Could you check a few things on this model? Use its own coordinates, in mm. Face numbers are marked on the shaded views. Round coordinates to 2 decimals unless told otherwise and drop trailing zeros. Write each loop counter-clockwise with the first axis right and the second up, starting at its lowest first coordinate (ties: lowest second). Pieces come first, ordered by that corner, then holes. Notation, with made-up numbers: M -14,81 L 7,81 A20 ccw 7,96 Z; hole C 12.25,-17 d8. An arc over 180 degrees is marked long. One line per question, with ' | ' between items. Start each with the question number.
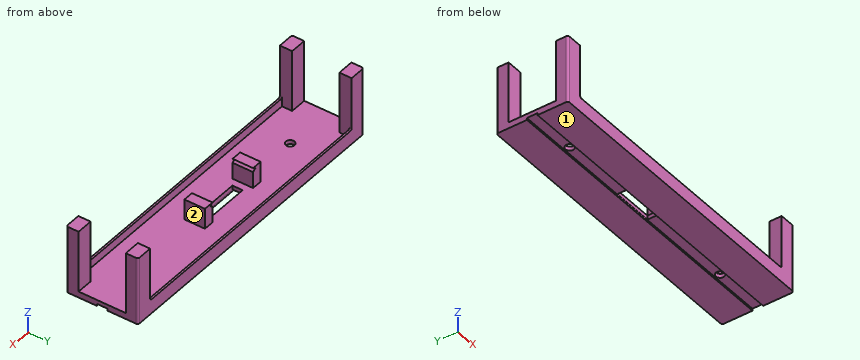
```python
from build123d import *

# Parameters (mm, degrees)
SKICA1_W                 = 150
SKICA1_H                 = 35
P_IDAT_VYSUNUT_M2_DEPTH  = 3
SKICA4_W                 = 20
SKICA4_H                 = 5
ODEBRAT_VYSUNUT_M1_DEPTH = 2
SKICA5_W                 = 150
SKICA5_H                 = 5.2
ODEBRAT_VYSUNUT_M3_DEPTH = 1
SKICA7_R                 = 2.1
ODEBRAT_VYSUNUT_M4_DEPTH = 3
SKICA8_W                 = 8
SKICA8_H                 = 6
P_IDAT_VYSUNUT_M4_DEPTH  = 30
ZAOBLIT1_R               = 1
SKICA9_W                 = 134
SKICA9_H                 = 1
P_IDAT_VYSUNUT_M5_DEPTH  = 4
ZAOBLIT2_R               = 1
SKICA10_W                = 5
SKICA10_H                = 10
P_IDAT_VYSUNUT_M6_DEPTH  = 10
ODEBRAT_VYSUNUT_M6_DEPTH = 10


with BuildPart() as part:
    # Skica1 → Přidat vysunutím2 (new body)
    with BuildSketch(Plane.XY):
        Rectangle(SKICA1_W, SKICA1_H)
    extrude(amount=P_IDAT_VYSUNUT_M2_DEPTH)

    # Skica4 → Odebrat vysunutím1 (cut)
    with BuildSketch(Plane.XY.offset(3)):
        with Locations((-5, 0)):
            Rectangle(SKICA4_W, SKICA4_H)
    extrude(amount=-ODEBRAT_VYSUNUT_M1_DEPTH, mode=Mode.SUBTRACT)

    # Skica5 → Odebrat vysunutím3 (cut)
    with BuildSketch(Plane(origin=(0, 0, 0), x_dir=(-1, 0, 0), z_dir=(0, 0, -1))):
        Rectangle(SKICA5_W, SKICA5_H)
    extrude(amount=-ODEBRAT_VYSUNUT_M3_DEPTH, mode=Mode.SUBTRACT)

    # Skica7 → Odebrat vysunutím4 (cut, through all)
    with BuildSketch(Plane(origin=(0, 0, 1), x_dir=(-1, 0, 0), z_dir=(0, 0, -1))):
        with Locations((-50, 0)):
            Circle(SKICA7_R)
        with Locations((50, 0)):
            Circle(SKICA7_R)
    extrude(amount=-ODEBRAT_VYSUNUT_M4_DEPTH, mode=Mode.SUBTRACT)

    # Skica8 → Přidat vysunutím4 (add)
    with BuildSketch(Plane.XY.offset(3)):
        with Locations((71, 14.5)):
            Rectangle(SKICA8_W, SKICA8_H)
        with Locations((71, -14.5)):
            Rectangle(SKICA8_W, SKICA8_H)
        with Locations((-71, -14.5)):
            Rectangle(SKICA8_W, SKICA8_H)
        with Locations((-71, 14.5)):
            Rectangle(SKICA8_W, SKICA8_H)
    extrude(amount=P_IDAT_VYSUNUT_M4_DEPTH)

    # Zaoblit1
    zaoblit1_edges = [part.edges().sort_by_distance(p)[0] for p in [
        (75, -17.5, 16.5),
        (75, 17.5, 16.5),
        (-75, 17.5, 16.5),
        (-75, -17.5, 16.5),
    ]]
    fillet(zaoblit1_edges, radius=ZAOBLIT1_R)

    # Skica9 → Přidat vysunutím5 (add)
    with BuildSketch(Plane.XY.offset(3)):
        with Locations((0, 17)):
            Rectangle(SKICA9_W, SKICA9_H)
        with Locations((0, -17)):
            Rectangle(SKICA9_W, SKICA9_H)
    extrude(amount=P_IDAT_VYSUNUT_M5_DEPTH)

    # Zaoblit2
    zaoblit2_edges = [part.edges().sort_by_distance(p)[0] for p in [
        (67, 17, 7),
        (-67, 17, 7),
        (-67, -17, 7),
        (67, -17, 7),
    ]]
    fillet(zaoblit2_edges, radius=ZAOBLIT2_R)

    # Skica10 → Přidat vysunutím6 (add)
    with BuildSketch(Plane.XY.offset(3)):
        with Locations((-21, 0)):
            Rectangle(SKICA10_W, SKICA10_H)
        with Locations((11, 0)):
            Rectangle(SKICA10_W, SKICA10_H)
    extrude(amount=P_IDAT_VYSUNUT_M6_DEPTH)

    # Skica12 → Odebrat vysunutím6 (cut)
    with BuildSketch(Plane(origin=(0, 5, 0), x_dir=(1, 0, 0), z_dir=(0, 1, 0))):
        Polygon((-18.5, -13), (-18.5, -11), (-20, -12), align=None)
        Polygon((8.5, -13), (8.5, -11), (10, -12), align=None)
    extrude(amount=-ODEBRAT_VYSUNUT_M6_DEPTH, mode=Mode.SUBTRACT)


solid = part.part
```
1. Suppose I cut it at B-B (x = -50). Write out the boundary of the cut face in (y, z), and give its area (3 significant figures).
2. Suppose I cut it at A-A (z = 20.5). Write out the boundary of the cut face in (x, y), and give its area (3 significant figures).
3. I'm going to push flat-ended pins straight in: P1, Ø4, axis at y = -2, z = 6.5, coming from the +X side; P2, Ø3, axis at x = 12.5, z = 10.5, coming from the -Y side; P3, Ø16.5, axis at x = 32, y = -4.5, coming from the +Z side. Where does each tip first touch, or does it pass through?
4. If we mould it in two halves opening along Y, with no side actions, what happens to the marked faces 1 and 2? For each: released by +Y, released by -Y, zero draft, split by the parting line, or undercut.
5. I need wall thicknesses on line 1 along Y through (x, z) = (21, 3.5); line 2 along Y through (x, z) = (-50, 2); line 3 along X through (y, z) = (-13.5, 20). Which ranges of each line are inside material? Lowest first, please. Write a range as from..to.
6. Suppose I cut it at D-D (x = -28.5). Write out the boundary of the cut face in (y, z), and give its area (3 significant figures).
7. Suppose I cut it at C-C (y = 0). Write out the boundary of the cut face in (x, z).
Computed:
1) outline: M -17.5,0 L -2.6,0 L -2.6,1 L -2.1,1 L -2.1,3 L -16.5,3 L -16.5,7 L -17.5,7 Z; M 2.1,1 L 2.6,1 L 2.6,0 L 17.5,0 L 17.5,7 L 16.5,7 L 16.5,3 L 2.1,3 Z | area: 99.4 mm²
2) outline: M -75,-16.5 A1 ccw -74,-17.5 L -67,-17.5 L -67,-11.5 L -75,-11.5 Z; M -75,11.5 L -67,11.5 L -67,17.5 L -74,17.5 A1 ccw -75,16.5 Z; M 67,-17.5 L 74,-17.5 A1 ccw 75,-16.5 L 75,-11.5 L 67,-11.5 Z; M 67,11.5 L 75,11.5 L 75,16.5 A1 ccw 74,17.5 L 67,17.5 Z | area: 191 mm²
3) P1: stops at x = 13.5 | P2: stops at y = -5 | P3: stops at z = 3
4) face 1: zero draft | face 2: undercut
5) line 1: y = -17.5..-16.5, 16.5..17.5 | line 2: y = -17.5..-2.1, 2.1..17.5 | line 3: x = -75..-67, 67..75
6) outline: M -17.5,0 L -2.6,0 L -2.6,1 L 2.6,1 L 2.6,0 L 17.5,0 L 17.5,7 L 16.5,7 L 16.5,3 L -16.5,3 L -16.5,7 L -17.5,7 Z | area: 108 mm²
7) outline: M -75,1 L -52.1,1 L -52.1,3 L -75,3 Z; M -47.9,1 L -15,1 L -15,3 L -18.5,3 L -18.5,11 L -20,12 L -18.5,13 L -23.5,13 L -23.5,3 L -47.9,3 Z; M 5,1 L 47.9,1 L 47.9,3 L 13.5,3 L 13.5,13 L 8.5,13 L 10,12 L 8.5,11 L 8.5,3 L 5,3 Z; M 52.1,1 L 75,1 L 75,3 L 52.1,3 Z
